Could you check a few things on this model? Use its own coordinates, in mm. A direction names the side the tool comes from. Give positions to 0.01 mm unless a question says otherwise; leave off trailing zeros. Order: outer loops, then holes, each group sorted by start corner. A loop starts at its lowest first (then second) coordinate and runs counter-clockwise, first axis right, second up. Notation, with made-up numbers: (54, -25) -> (87, -25) arc R26 cw to (87, -6) -> close; hole circle Ø10 at (38, -19.75). An arc over 180 degrees is marked (long way). Use one line per item in the form item = value. Start each with the question number.
from build123d import *

# Parameters (mm, degrees)
F0_W     = 23.253381
F0_H     = 83.83457
F1_DEPTH = 72.898
F2_R     = 7.595409
F3_DEPTH = 112.014
F4_W     = 61.105391
F4_H     = 29.362335
F5_DEPTH = 109.982


with BuildPart() as f1:
    # F0 (on Top) → F1 (new body)
    with BuildSketch(Plane.XY):
        Polygon((-68.383306, -55.073805), (-68.383306, -66.700496), (55.226788, -66.700496), (55.226788, -55.073805), (33.809196, -55.073805), (-45.129925, -55.073805), align=None)
        with Locations((-56.756615, -13.15652)):
            Rectangle(F0_W, F0_H)
        Polygon((-68.383306, 52.01415), (-68.383306, 28.760765), (-45.129925, 28.760765), (33.809196, 28.760765), (33.809196, 52.01415), align=None)
        Polygon((33.809196, -55.073805), (55.226788, -55.073805), (55.226788, 52.01415), (33.809196, 52.01415), (33.809196, 28.760765), align=None)
    extrude(amount=F1_DEPTH)

    # F2 (on Front) → F3 (cut, symmetric)
    with BuildSketch(Plane.XZ):
        with Locations((0, 37.939731)):
            Circle(F2_R)
    extrude(amount=F3_DEPTH, both=True, mode=Mode.SUBTRACT)

    # F4 (on Right) → F5 (cut, symmetric)
    with BuildSketch(Plane.YZ):
        with Locations((-8.457915, 59.161521)):
            Rectangle(F4_W, F4_H)
    extrude(amount=F5_DEPTH, both=True, mode=Mode.SUBTRACT)


solid = f1.part
(1) I'm going to push flat-ended pins straight in: pin 1 Ø12 at (x, z) = (0, 37.94) entering from -Y; pin 2 Ø23.5 at (x, y) = (43, -3) entering from +Z. Where does each tip first touch, or does it pass through?
(2) Imagine slicing it at A-A (x = 0). Write out the boundary of the cut face in (y, z), plus the area to 3 significant figures.
(3) Imagine slicing it at B-B (y = -52.5). Write out the boundary of the cut face in (x, z), plus the area to 3 significant figures.
(4) Please list where these lines run through material, in increasing order: probe 1 along X at (y, z) = (28, 4.5); probe 2 along Y at (x, z) = (-19, 55); probe 3 along Y at (x, z) = (-49, 45.5).
(5) Imagine slicing it at D-D (x = 23.5). Write out the boundary of the cut face in (y, z).
(6) We'd pull the mould along X, two halves only. Please class faces 1 (the flat face through (-5, -55.074, 28)), 2 (the flat face through (-7, 33, 0)), 3 (the flat face through (-68.383, -61, 36)): pulls with the +X half, pulls with the -X half, needs draft (parallel to the pull), parting line crosses it, or undercut.
(7) Imagine slicing it at C-C (z = 52.5). Write out the boundary of the cut face in (x, y), plus the area to 3 significant figures.
(8) Which directions (+Z, -Z, +X, -X, +Y, -Y) give clear straight access to the entire face, cutting with the end or side of a thin tool? Please do faces 4 (the flat face through (55.227, -8, 28)), 5 (the flat face through (-57, -9, 44.48)), 6 (the flat face through (-6, 28.761, 28)).
Calculated:
q1.pin_1 = through
q1.pin_2 = 44.48
q2.outline = (-66.7, 0) -> (-55.07, 0) -> (-55.07, 30.34) -> (-66.7, 30.34) -> close; (-66.7, 45.54) -> (-55.07, 45.54) -> (-55.07, 72.9) -> (-66.7, 72.9) -> close; (28.76, 0) -> (52.01, 0) -> (52.01, 30.34) -> (28.76, 30.34) -> close; (28.76, 45.54) -> (52.01, 45.54) -> (52.01, 72.9) -> (28.76, 72.9) -> close
q2.area = 2,010 mm2
q3.outline = (-68.38, 0) -> (-45.13, 0) -> (-45.13, 72.9) -> (-68.38, 72.9) -> close; (33.81, 0) -> (55.23, 0) -> (55.23, 72.9) -> (33.81, 72.9) -> close
q3.area = 3,260 mm2
q4.probe_1 = -68.38 to -45.13, 33.81 to 55.23
q4.probe_2 = -66.7 to -55.07, 28.76 to 52.01
q4.probe_3 = -66.7 to -39.01, 22.09 to 52.01
q5.outline = (-66.7, 0) -> (-55.07, 0) -> (-55.07, 72.9) -> (-66.7, 72.9) -> close; (28.76, 0) -> (52.01, 0) -> (52.01, 72.9) -> (28.76, 72.9) -> close
q6.face_1 = undercut
q6.face_2 = needs draft
q6.face_3 = pulls with the -X half
q7.outline = (-68.38, -66.7) -> (55.23, -66.7) -> (55.23, -39.01) -> (33.81, -39.01) -> (33.81, -55.07) -> (-45.13, -55.07) -> (-45.13, -39.01) -> (-68.38, -39.01) -> close; (-68.38, 22.09) -> (-45.13, 22.09) -> (-45.13, 28.76) -> (33.81, 28.76) -> (33.81, 22.09) -> (55.23, 22.09) -> (55.23, 52.01) -> (-68.38, 52.01) -> close
q7.area = 5,330 mm2
q8.face_4 = +Z, -Z, +X, +Y, -Y
q8.face_5 = +Z, +X, -X
q8.face_6 = +Z, -Z
